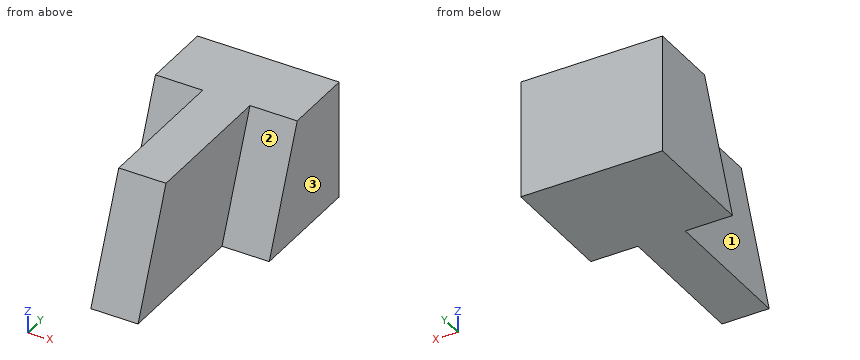
```python
from build123d import *

# Parameters (mm, degrees)
F1_DEPTH = 31.75
F3_DEPTH = 25.4
F5_DEPTH = 12.7
F7_DEPTH = 12.7


with BuildPart() as f1:
    # F0 (on Top) → F1 (new body)
    with BuildSketch(Plane.XY):
        Polygon((0, 38.1), (0, 0), (12.7, 0), (12.7, 38.1), (25.4, 38.1), (25.4, 69.85), (-12.7, 69.85), (-12.7, 38.1), align=None)
    extrude(amount=F1_DEPTH)

    # F2 (on face) → F3 (cut)
    with BuildSketch(Plane(origin=(0, 0, 0), x_dir=(0, -1, 0), z_dir=(-1, 0, 0))):
        Polygon((0, 0), (0, 31.75), (-12.7, 31.75), align=None)
    extrude(amount=-F3_DEPTH, mode=Mode.SUBTRACT)

    # F4 (on face) → F5 (cut)
    with BuildSketch(Plane(origin=(-12.7, 0, 0), x_dir=(0, -1, 0), z_dir=(-1, 0, 0))):
        Polygon((-38.1, 0), (-38.1, 31.75), (-50.8, 31.75), align=None)
    extrude(amount=-F5_DEPTH, mode=Mode.SUBTRACT)

    # F6 (on face) → F7 (cut)
    with BuildSketch(Plane.YZ.offset(25.4)):
        Polygon((50.8, 31.75), (38.1, 31.75), (38.1, 0), align=None)
    extrude(amount=-F7_DEPTH, mode=Mode.SUBTRACT)


solid = f1.part
```
The model under review builds one solid part; all positions refer to its coordinate system, in mm. Face numbers are marked on the shaded views. A direction names the side the tool comes from. Round coordinates to 2 decimals unless told otherwise and drop trailing zeros. Loops run counter-clockwise (first coordinate to the right, second up) from the corner with the lowest first, then second, coordinate; pieces in that order, holes last. Notation, with made-up numbers: (79, 83.25) -> (124, 83.25) arc R35 cw to (124, 118.25) -> close; hole circle Ø5 at (71.5, -12.5). An arc over 180 degrees is marked (long way). Answer in a Markdown table with one row per item.
1) Tool access review of the marked faces 1, 2 and 3: name each direction out of +Z, -Z, +X, -X, +Y, -Y from which nothing blocks a thin tool from reaching the whole face with its end or side.
Taken from the geometry:
| item | result |
|---|---|
| face 1 | +Z, -X, -Y |
| face 2 | +Z, +X, -Y |
| face 3 | +Z, -Z, +X, +Y, -Y |
2) Consider section B-B, the plane z = 18. Write out the cut boundary in (x, y), plus the area to 3 significant figures.
Taken from the geometry:
| item | result |
|---|---|
| outline | (-12.7, 45.3) -> (0, 45.3) -> (0, 7.2) -> (12.7, 7.2) -> (12.7, 45.3) -> (25.4, 45.3) -> (25.4, 69.85) -> (-12.7, 69.85) -> close |
| area | 1,420 mm² |
3) Consider section C-C, the plane x = 17. Write out the cut boundary in (y, z).
Taken from the geometry:
| item | result |
|---|---|
| outline | (38.1, 0) -> (69.85, 0) -> (69.85, 31.75) -> (50.8, 31.75) -> close |
4) Wall thickness on line 1 along X through (y, z) = (29, 20); line 2 along Y through (x, z) = (4, 23); line 3 along Y through (x, z) = (-1, 9.5): over which ranges is each line inside the solid? List them lowest first.
Taken from the geometry:
| item | result |
|---|---|
| line 1 | x = 0 to 12.7 |
| line 2 | y = 9.2 to 69.85 |
| line 3 | y = 41.9 to 69.85 |
5) For pin 1 Ø4 at (x, z) = (7.5, 6) entering from -Y; pin 2 Ø4 at (x, z) = (12, 5.5) entering from -Y; pin 3 Ø4 at (x, y) = (14, 27.5) entering from +Z; pin 4 Ø3 at (x, z) = (-3, 16) entering from -Y, all flat-tipped, find the tip position at first contact; note any pin that passes through.
Taken from the geometry:
| item | result |
|---|---|
| pin 1 | stops at y = 1.6 |
| pin 2 | stops at y = 1.4 |
| pin 3 | stops at z = 31.75 |
| pin 4 | stops at y = 43.9 |
6) Consider section D-D, the plane y = 24. Write out the cut boundary in (x, z), plus the area to 3 significant figures.
Taken from the geometry:
| item | result |
|---|---|
| outline | (0, 0) -> (12.7, 0) -> (12.7, 31.75) -> (0, 31.75) -> close |
| area | 403 mm² |
7) Consider section A-A, the plane y = 40. Write out the cut boundary in (x, z).
Taken from the geometry:
| item | result |
|---|---|
| outline | (-12.7, 0) -> (25.4, 0) -> (25.4, 4.75) -> (12.7, 4.75) -> (12.7, 31.75) -> (0, 31.75) -> (0, 4.75) -> (-12.7, 4.75) -> close |
